```python
from build123d import *

# Parameters (mm, degrees)
EXTRUDE2_START     = -11.1125
EXTRUDE2_OUTLINE_R = 7.9375
EXTRUDE2_DEPTH     = 22.225
SKETCH2_W          = 762
SKETCH2_H          = 63.5
EXTRUDE3_DEPTH     = 279.4


# Read off the part's stored shape, not the designer's step: Extrude2
with BuildPart() as part:
    # Extrude2 outline → Extrude2 (new body)
    with BuildSketch(Plane.XY.offset(EXTRUDE2_START)):
        with BuildLine():
            ThreePointArc((55.379666285, 831.639308698), (87.129666285, 799.889308698), (118.879666285, 831.639308698))
            Line((118.879666285, 831.639308698), (118.879666285, 867.199308698))
            Line((118.879666285, 867.199308698), (55.379666285, 867.199308698))
            Line((55.379666285, 867.199308698), (55.379666285, 831.639308698))
        make_face()
        with Locations((87.129666285, 831.639308698)):
            Circle(EXTRUDE2_OUTLINE_R, mode=Mode.SUBTRACT)
    extrude(amount=EXTRUDE2_DEPTH)

    # Sketch2 → Extrude3 (add, symmetric)
    with BuildSketch(Plane.XY):
        with Locations((87.129666285, 898.949308698)):
            Rectangle(SKETCH2_W, SKETCH2_H)
    extrude(amount=EXTRUDE3_DEPTH, both=True)


solid = part.part
```
Read the model definition and answer for the solid it produces. Units are mm, in the model's axes. A direction names the side the tool comes from. Coordinates: 2 decimals unless noted, no trailing zeros. Loops run counter-clockwise (first coordinate to the right, second up) from the corner with the lowest first, then second, coordinate; pieces in that order, holes last.
(1) The part is cut by section C-C (x = 69.5). Determine the outline of the cut face in (y, z).
Solution:
outline: (805.23, -11.11) - (867.2, -11.11) - (867.2, -279.4) - (930.7, -279.4) - (930.7, 279.4) - (867.2, 279.4) - (867.2, 11.11) - (805.23, 11.11) - close
(2) The mould has two halves that part along Y. Classify faces 6 (the face through (82, 899, 279.4)), 7 (the face through (86.432, 799.897, -0.156)), 8 (the face through (86.1, 839.51, -0.16)), 9 (the face through (82, 930.699, 4)): released by +Y, released by -Y, zero draft, split by the parting line, or undercut.
Solution:
face 6: zero draft
face 7: released by -Y
face 8: undercut
face 9: released by +Y
(3) The part is cut by section B-B (x = 202). Determine the outline of the cut face in (y, z), and give its area (3 significant figures).
Solution:
outline: (867.2, -279.4) - (930.7, -279.4) - (930.7, 279.4) - (867.2, 279.4) - close
area: 35,500 mm2
(4) A tool of negligible diameter and unlimited length cuts with its end or side. For faces 1 (the face through (87, 841, -11.112)), 2 (the face through (118.88, 849, 0)), 3 (the face through (87, 841, 11.112)), 4 (the face through (-293.87, 899, 4)), 5 (the face through (55.38, 850, 0)), from which of +Z, -Z, +X, -X, +Y, -Y can it reach the whole face along a straight path? Write none if from no direction.
Solution:
face 1: -Z, +X, -X, -Y
face 2: +Z, -Z, +X, -Y
face 3: +Z, +X, -X, -Y
face 4: +Z, -Z, -X, +Y, -Y
face 5: +Z, -Z, -X, -Y
(5) Consider line 1 along Y through (x, z) = (-39, 102); line 2 along Z through (x, y) = (103, 813). Determine where each line is inside the solid, lowest interval first.
Solution:
line 1: y = 867.2 to 930.7
line 2: z = -11.11 to 11.11
(6) Flat-ended cylindrical pins translate along their axes: pin 1 Ø4 at (x, z) = (-48.5, -169.5) entering from -Y; pin 2 Ø6.5 at (y, z) = (843, -4) entering from -X; pin 3 Ø18 at (y, z) = (848, -5) entering from +X. Find the tip coordinate at first contact, or state that the pin passes through.
Solution:
pin 1: stops at y = 867.2
pin 2: stops at x = 55.38
pin 3: stops at x = 118.88
(7) The part is cut by section A-A (z = -137.5). Determine the outline of the cut face in (x, y).
Solution:
outline: (-293.87, 867.2) - (468.13, 867.2) - (468.13, 930.7) - (-293.87, 930.7) - close
